Check sheet for the modelled part. Datum: model origin and axes. Units: mm. A direction names the side the tool comes from. Coordinates: 2 decimals unless noted, no trailing zeros. Loops run counter-clockwise (first coordinate to the right, second up) from the corner with the lowest first, then second, coordinate; pieces in that order, holes last. Notation, with made-up numbers: M 10.25,-33.5 L 54.25,-33.5 A27 cw 54.25,-2.5 Z; hole C -16.75,34 d8. An arc over 180 degrees is marked long. Use CSV: the item, a comma, the result in double quotes. Start each with the question number.
(1) Scan lines: line 1 (X direction, y = 4, z = 4.5); line 2 (Y direction, x = 17.75, z = 4.55); line 3 (Y direction, x = 8.75, z = 0.7). Record each from-to range of solid material in increasing order.
(2) Section check C-C on z = 3.6. Record the cut outline in (x, y), and give its area (3 significant figures).
(3) Section check A-A on y = 20. Record the cut outline in (x, z), and give its area (3 significant figures).
(4) Section check D-D on z = 0.85. Record the cut outline in (x, y), and give its area (3 significant figures).
(5) Section check B-B on x = 19. Record the cut outline in (y, z).
(6) Draft check along X on faces 5 (the flat face through (2, 20, 4)), 6 (the flat face through (22.5, 20, 3)), 7 (the flat face through (2, 0, 3)). Enter one of: pulls with the +X half, pulls with the -X half, needs draft (parallel to the pull), parting line crosses it, or undercut.
(7) Set-up check for faces 1 (the flat face through (18.5, 21, 1)), 2 (the flat face through (11, 38, 3)), 3 (the flat face through (11, 40, 3)), 4 (the flat face through (17.5, 1.5, 2.4)): record each of +Z, -Z, +X, -X, +Y, -Y from which the full face is reachable in a straight line by a thin tool's end or side.
(8) Go/stop test with flat-tipped pins: pin 1 Ø2 at (x, z) = (14.5, 3.5) entering from -Y; pin 2 Ø2.5 at (x, y) = (3, 14) entering from +Z; pin 3 Ø1 at (x, y) = (19, 7.5) entering from +Z. Record where each tip stops, or that it passes through.
from build123d import *

# Parameters (mm, degrees)
SKETCH064_W         = 22.5
SKETCH064_H         = 40
PAD034_DEPTH        = 6
SKETCH065_W         = 18.5
SKETCH065_H         = 36
POCKET020_DEPTH     = 4
SKETCH062_W         = 14.5
SKETCH062_H         = 32
POCKET021_DEPTH     = 2.001
SKETCH063_W         = 12.5
SKETCH063_H         = 4
POCKET022_DEPTH     = 6.001
REVOLUTION005_ANGLE = -180
REVOLUTION006_ANGLE = 180
SKETCH084_W         = 14.5
SKETCH084_H         = 2
POCKET029_DEPTH     = 2.001


with BuildPart() as part:
    # Sketch064 → Pad034 (new body)
    with BuildSketch(Plane.XY):
        with Locations((11.25, 20)):
            Rectangle(SKETCH064_W, SKETCH064_H)
    extrude(amount=PAD034_DEPTH)

    # Sketch065 (on Face6 of Pad034) → Pocket020 (cut)
    with BuildSketch(Plane.XY.offset(6)):
        with Locations((11.25, 20)):
            Rectangle(SKETCH065_W, SKETCH065_H)
    extrude(amount=-POCKET020_DEPTH, mode=Mode.SUBTRACT)

    # Sketch062 (on Face11 of Pocket020) → Pocket021 (cut, through all)
    with BuildSketch(Plane.XY.offset(2)):
        with Locations((11.25, 20)):
            Rectangle(SKETCH062_W, SKETCH062_H)
    extrude(amount=-POCKET021_DEPTH, mode=Mode.SUBTRACT)

    # Sketch063 (on Face5 of Pocket021) → Pocket022 (cut, through all)
    with BuildSketch(Plane.XY.offset(6)):
        with Locations((11.25, 2)):
            Rectangle(SKETCH063_W, SKETCH063_H)
    extrude(amount=-POCKET022_DEPTH, mode=Mode.SUBTRACT)

    # Sketch067 (on Face20 of Pocket022) → Revolution005 (revolve)
    with BuildSketch(Plane.YZ.offset(2)):
        with BuildLine():
            ThreePointArc((14, 5), (13, 6), (12, 5))
            Line((12, 5), (14, 5))
        make_face()
        with BuildLine():
            ThreePointArc((33, 5), (32, 6), (31, 5))
            Line((31, 5), (33, 5))
        make_face()
    revolve(axis=Axis((2, 14, 5), (0, -1, 0)), revolution_arc=REVOLUTION005_ANGLE)

    # Sketch068 (on Face19 of Revolution005) → Revolution006 (revolve)
    with BuildSketch(Plane(origin=(20.5, 0, 0), x_dir=(0, -1, 0), z_dir=(-1, 0, 0))):
        with BuildLine():
            ThreePointArc((-31, 5), (-32, 6), (-33, 5))
            Line((-33, 5), (-31, 5))
        make_face()
        with BuildLine():
            ThreePointArc((-12, 5), (-13, 6), (-14, 5))
            Line((-14, 5), (-12, 5))
        make_face()
    revolve(axis=Axis((20.5, 31, 5), (0, -1, 0)), revolution_arc=REVOLUTION006_ANGLE)

    # Sketch084 (on Face15 of Revolution006) → Pocket029 (cut, through all)
    with BuildSketch(Plane.XY.offset(2)):
        with Locations((11.25, 37)):
            Rectangle(SKETCH084_W, SKETCH084_H)
    extrude(amount=-POCKET029_DEPTH, mode=Mode.SUBTRACT)


solid = part.part
Outcome:
1,line 1,"x = 0 to 2, 20.5 to 22.5"
1,line 2,"y = 0 to 2, 38 to 40"
1,line 3,"y = 38 to 40"
2,outline,"M 0,0 L 5,0 L 5,2 L 2,2 L 2,38 L 20.5,38 L 20.5,2 L 17.5,2 L 17.5,0 L 22.5,0 L 22.5,40 L 0,40 Z"
2,area,"209 mm²"
3,outline,"M 0,0 L 4,0 L 4,2 L 2,2 L 2,6 L 0,6 Z; M 18.5,0 L 22.5,0 L 22.5,6 L 20.5,6 L 20.5,2 L 18.5,2 Z"
3,area,"32.0 mm²"
4,outline,"M 0,0 L 5,0 L 5,4 L 4,4 L 4,38 L 18.5,38 L 18.5,4 L 17.5,4 L 17.5,0 L 22.5,0 L 22.5,40 L 0,40 Z"
4,area,"357 mm²"
5,outline,"M 0,0 L 40,0 L 40,6 L 38,6 L 38,2 L 2,2 L 2,6 L 0,6 Z"
6,face 5,"undercut"
6,face 6,"pulls with the +X half"
6,face 7,"needs draft"
7,face 1,"+Z, -Z"
7,face 2,"+Z"
7,face 3,"+Z, -Z, +X, -X, +Y"
7,face 4,"+Z, -Z, -Y"
8,pin 1,"stops at y = 38"
8,pin 2,"stops at z = 6"
8,pin 3,"stops at z = 2"
